Source: CAD feature listing. Evaluate the final solid. Frame: model axes, mm. A direction names the side the tool comes from. Coordinates: 2 decimals unless noted, no trailing zeros. Loops run counter-clockwise (first coordinate to the right, second up) from the corner with the lowest first, then second, coordinate; pieces in that order, holes last.
from build123d import *

# Parameters (mm, degrees)
BOSS_EXTRUDE1_DEPTH = 500
CUT_EXTRUDE1_DEPTH  = 70
CUT_EXTRUDE2_DEPTH  = 35
FILLET1_R           = 10
SKETCH4_R           = 12.5
CUT_EXTRUDE3_DEPTH  = 70


with BuildPart() as part:
    # Sketch1 → Boss-Extrude1 (new, symmetric)
    with BuildSketch(Plane.XY):
        Polygon((-14.024390244, 39.268292683), (-9.024390244, 39.268292683), (-9.024390244, -5.731707317), (35.975609756, -5.731707317), (35.975609756, -10.731707317), (-14.024390244, -10.731707317), align=None)
    extrude(amount=BOSS_EXTRUDE1_DEPTH, both=True)

    # Sketch2 → Cut-Extrude1 (cut)
    with BuildSketch(Plane(origin=(0, 39.268292683, 0), x_dir=(1, 0, 0), z_dir=(0, 1, 0))):
        with BuildLine():
            Line((-62.224317274, 529.897722978), (58.968835914, 529.897722978))
            Line((58.968835914, 529.897722978), (58.968835914, 344.739681267))
            ThreePointArc((58.968835914, 344.739681267), (0.874290628, 380.84092237), (-62.224317274, 407.238677616))
            Line((-62.224317274, 407.238677616), (-62.224317274, 529.897722978))
        make_face()
        with BuildLine():
            Line((75.729591142, -524.740567523), (-50.6207175, -524.740567523))
            Line((-50.6207175, -524.740567523), (-50.6207175, -403.255719892))
            ThreePointArc((-50.6207175, -403.255719892), (8.569896952, -376.772838636), (63.086584035, -341.661548879))
            Line((63.086584035, -341.661548879), (75.729591142, -341.661548879))
            Line((75.729591142, -341.661548879), (75.729591142, -524.740567523))
        make_face()
    extrude(amount=-CUT_EXTRUDE1_DEPTH, mode=Mode.SUBTRACT)

    # Sketch3 → Cut-Extrude2 (cut, symmetric)
    with BuildSketch(Plane(origin=(-9.024390244, 0, 0), x_dir=(0, 0, -1), z_dir=(1, 0, 0))):
        Polygon((388.162337174, -10.731707317), (328.162337174, 39.268292683), (388.162337174, 39.268292683), align=None)
    cut_extrude2 = extrude(amount=CUT_EXTRUDE2_DEPTH, both=True, mode=Mode.SUBTRACT)

    # Mirror1: Cut-Extrude2 across plane
    add(cut_extrude2.mirror(Plane.XY), mode=Mode.SUBTRACT)

    # Fillet1
    fillet1_edges = [part.edges().sort_by_distance(p)[0] for p in [
        (-11.524390244, 39.268292683, -328.162337174),
        (-11.524390244, 39.268292683, 328.162337174),
    ]]
    fillet(fillet1_edges, radius=FILLET1_R)

    # Sketch4 → Cut-Extrude3 (cut)
    with BuildSketch(Plane(origin=(-9.024390244, 0, 0), x_dir=(0, 0, -1), z_dir=(1, 0, 0))):
        with Locations(Location((318.162337174, 16.268292683, 0), (0, 0, 90))):
            Circle(SKETCH4_R)
        with Locations(Location((-318.162337174, 16.268292683, 0), (0, 0, 90))):
            Circle(SKETCH4_R)
    extrude(amount=-CUT_EXTRUDE3_DEPTH, mode=Mode.SUBTRACT)


solid = part.part
Q1. Contact query for flat-ended pins moving along their axis: pin 1 Ø10 at (x, z) = (14.5, 27) entering from +Y; pin 2 Ø1 at (y, z) = (3.5, 209) entering from +X. Output: stop coordinate, or through.
Q2. Section B-B, the plane z = 85.5. Return the cut outline in (x, y), plus the area to 3 significant figures.
Q3. Draft query along Y for faces 3 (the cylindrical face through (-11.49, 22.04, -329.25)), 4 (the flat face through (11, -10.732, 5)), 5 (the cylindrical face through (-11.489, 22.036, 307.073)), 6 (the flat face through (13, -5.732, 5)). Return one class per face: +Y half, -Y half, draft (parallel to the pull), parting line (faces both ways), or undercut.
Q4. Section C-C, the plane x = 12. Return the cut outline in (y, z).
Q5. Section A-A, the plane y = 20. Return the cut outline in (x, z).
Q6. Access query for faces 1 (the flat face through (-10.52, 12.78, 359.95)), 2 (the flat face through (-9.024, 17, 5)). Directions: +Z, -Z, +X, -X, +Y, -Y. A direction counts if a zero-diameter tool reaches every point of the face in a straight line with its end or side. Return the directions, or none.
Q7. Line query: line 1 along Y through (x, z) = (7, -41.5); line 2 along X through (y, z) = (4.5, 96); line 3 along Z through (x, y) = (-11, 2). Output: solid intervals per line, ascending.
Derived:
1. pin 1: stops at y = -5.73
1. pin 2: stops at x = -9.02
2. outline: (-14.02, -10.73) - (35.98, -10.73) - (35.98, -5.73) - (-9.02, -5.73) - (-9.02, 39.27) - (-14.02, 39.27) - close
2. area: 475 mm2
3. face 3: undercut
3. face 4: -Y half
3. face 5: undercut
3. face 6: +Y half
4. outline: (-10.73, -374.89) - (-5.73, -374.89) - (-5.73, 374.89) - (-10.73, 374.89) - close
5. outline: (-14.02, -351.28) - (-9.02, -351.28) - (-9.02, -330.09) - (-14.02, -330.09) - close; (-14.02, -306.23) - (-9.02, -306.23) - (-9.02, 306.23) - (-14.02, 306.23) - close; (-14.02, 330.09) - (-9.02, 330.09) - (-9.02, 351.28) - (-14.02, 351.28) - close
6. face 1: +Z, +X, -X, +Y
6. face 2: +Z, -Z, +X, +Y
7. line 1: y = -10.73 to -5.73
7. line 2: x = -14.02 to -9.02
7. line 3: z = -372.88 to 372.88
